```python
from build123d import *

# Parameters (mm, degrees)
F0_R     = 10.9982
F1_DEPTH = 6.35


# Not quite as in the source:
# - a feature names something its author has since deleted; it is built from what else it names


with BuildPart() as f1:
    # F0 (on Top) → F1 (new body)
    with BuildSketch(Plane.XY):
        with BuildLine():
            ThreePointArc((23.5712, -34.728333354), (19.5070052041, -0.0046640159), (23.674090089, 34.706808082))
            ThreePointArc((23.674090089, 34.706808082), (0.1039423202, 58.2769558508), (-23.4662054486, 34.706808082))
            ThreePointArc((-23.4662054486, 34.706808082), (-19.3723117522, -0.1418189062), (-23.569876554, -34.9781105903))
            ThreePointArc((-23.569876554, -34.9781105903), (0.1248903712, -58.2992024902), (23.5712, -34.728333354))
        make_face()
        with Locations((0, -34.728333354)):
            Circle(F0_R, mode=Mode.SUBTRACT)
        Circle(F0_R, mode=Mode.SUBTRACT)
        with Locations((0.1039423202, 34.706808082)):
            Circle(F0_R, mode=Mode.SUBTRACT)
    extrude(amount=F1_DEPTH)


solid = f1.part
```
Verification items for the finished model (mm, model axes). Give positions to 0.01 mm unless a question says otherwise; leave off trailing zeros. Order: outer loops, then holes, each group sorted by start corner. A loop starts at its lowest first (then second) coordinate and runs counter-clockwise, first axis right, second up. Notation, with made-up numbers: M -39.75,4 L -15.75,4 A28 ccw -15.75,23 Z; hole C 83,20 d11. An arc over 180 degrees is marked long. Return JSON: item names as keys, results as strings. Group by question number.
1) Go/stop test with flat-tipped pins: pin 1 Ø20 at (x, y) = (0.1, 34.71) entering from +Z; pin 2 Ø3 at (x, z) = (-3, 5.5) entering from -Y; pin 3 Ø1.5 at (x, z) = (10, 5.5) entering from +Y; pin 4 Ø5 at (x, y) = (5, -25.5) entering from +Z. Record where each tip stops, or that it passes through.
2) Section check C-C on x = -4. Record the cut outline in (y, z).
3) Section check D-D on y = 37.5. Record the cut outline in (x, z), and give its area (3 significant figures).
4) Section check B-B on y = -33. Record the cut outline in (x, z).
5) Section check A-A on z = 1.75. Record the cut outline in (x, y).
6) Mould release check, pull along Y, two halves, no side actions. Record for faces 1 (the face through (-19.372, 0.351, 3.131)), 2 (the face through (0, -12, 6.35)), 3 (the face through (-0.392, -58.296, 3.131)): pulls with the +Y half, pulls with the -Y half, needs draft (parallel to the pull), parting line crosses it, or undercut.
7) Scan lines: line 1 (Y direction, x = 0, z = 4.5); line 2 (Y direction, x = -8, z = 5.5); line 3 (X direction, y = -4.5, z = 3.75). Record each from-to range of solid material in increasing order.
Answer block:
{
 "1": {"pin 1": "passes through", "pin 2": "stops at y = -58.25", "pin 3": "stops at y = 56.43", "pin 4": "stops at z = 6.35"},
 "2": {"outline": "M -57.96,0 L -44.97,0 L -44.97,6.35 L -57.96,6.35 Z; M -24.48,0 L -10.25,0 L -10.25,6.35 L -24.48,6.35 Z; M 10.25,0 L 24.5,0 L 24.5,6.35 L 10.25,6.35 Z; M 44.91,0 L 57.92,0 L 57.92,6.35 L 44.91,6.35 Z"},
 "3": {"outline": "M -23.3,0 L -10.53,0 L -10.53,6.35 L -23.3,6.35 Z; M 10.74,0 L 23.51,0 L 23.51,6.35 L 10.74,6.35 Z", "area": "162 mm^2"},
 "4": {"outline": "M -23.1,0 L -10.86,0 L -10.86,6.35 L -23.1,6.35 Z; M 10.86,0 L 23.17,0 L 23.17,6.35 L 10.86,6.35 Z"},
 "5": {"outline": "M -23.57,-34.98 A23.57 ccw 23.57,-34.73 A148.49 cw 23.67,34.71 A23.57 ccw -23.47,34.71 A148.49 cw Z; hole C 0,-34.73 d22; hole C 0,0 d22; hole C 0.1,34.71 d22"},
 "6": {"face 1": "undercut", "face 2": "needs draft", "face 3": "pulls with the -Y half"},
 "7": {"line 1": "y = -58.3 to -45.73, -23.73 to -11, 11 to 23.71, 45.7 to 58.28", "line 2": "y = -56.9 to -42.28, -27.18 to -7.55, 7.55 to 27.27, 42.14 to 56.84", "line 3": "x = -19.44 to -10.04, 10.04 to 19.57"}
}
